The drawing under review shows one solid part. Ordinate dimensions are in mm from its lowest x, y, z. A direction names the side the tool comes from. Coordinates: 2 decimals unless noted, no trailing zeros. Write each loop counter-clockwise with the first axis right and the second up, starting at its lowest first coordinate (ties: lowest second). Pieces come first, ordered by that corner, then holes. Notation, with made-up numbers: (16, -9) - (28, -9) arc R28 ccw to (28, 18) - close; hole circle Ø9 at (49, 34.25). An arc over 180 degrees is marked (long way). Put each result on its own line as item: value. Start each with the question number.
Item 1: Mouldability with a two-part tool opening along X and no side actions: class the marked faces 1, 2, 3 and 4 as pulls with the +X half, pulls with the -X half, needs draft (parallel to the pull), parting line crosses it, or undercut.
Item 2: Consider section A-A on x = 10. Give the boundary of the cut face in (y, z), then the cut area to 3 significant figures.
Item 3: For pin 1 (2 mm diameter, centred on x = 14.5, y = 3.5, fed in from -Z); pin 2 (12 mm diameter, centred on y = 16.5, z = 20.5, fed in from -X); pin 3 (12 mm diameter, centred on x = 10, z = 22.5, fed in from +Y), all flat-tipped, find the tip position at first contact; note any pin that passes through.
Item 4: Consider section D-D on z = 20.5. Give the boundary of the cut face in (x, y), then the cut area to 4 significant figures.
Item 5: Consider section C-C on y = 12.5. Give the boundary of the cut face in (x, z), then the cut area to 3 significant figures.
Item 6: Consider section B-B on z = 4.25. Give the boundary of the cut face in (x, y), then the cut area to 3 significant figures.
Item 7: To check wall thickness, follow L1, parallel to Z at x = 12.5, y = 10; L2, parallel to X at y = 10, z = 4.5; L3, parallel to Z at x = 17.5, y = 7.75. State the ranges of each line that lie inside material, in increasing order. Write a range as [from, to].
Item 8: Machinability: for the marked faces 5, 6, 7, 8 and 9, which of the approach directions +Z, -Z, +X, -X, +Y, -Y give a long, thin tool a straight path to every point of the face, cutting with its end or side? Answer none if there is none.
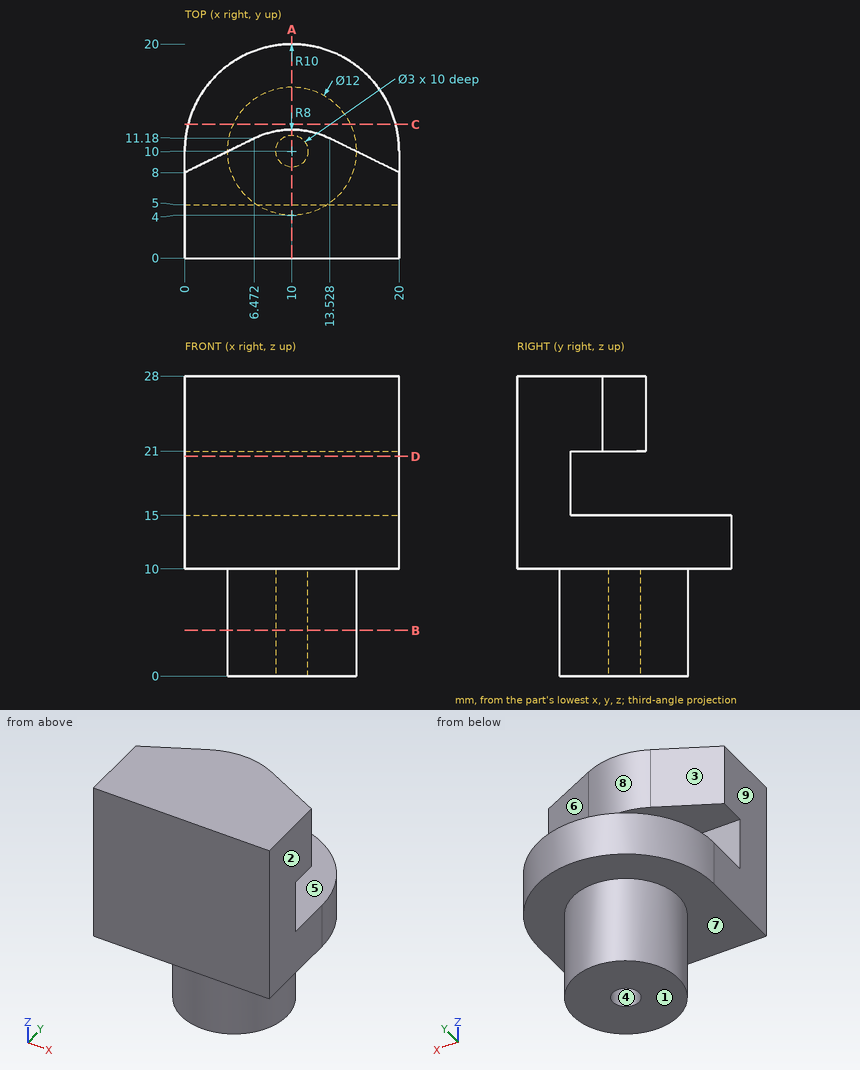
Report:
1. face 1: needs draft
1. face 2: pulls with the +X half
1. face 3: pulls with the -X half
1. face 4: undercut
2. outline: (0, 10) - (4, 10) - (4, 0) - (8.5, 0) - (8.5, 10) - (11.5, 10) - (11.5, 0) - (16, 0) - (16, 10) - (20, 10) - (20, 15) - (5, 15) - (5, 21) - (12, 21) - (12, 28) - (0, 28) - close
2. area: 304 mm²
3. pin 1: z = 10
3. pin 2: x = 0.88
3. pin 3: y = 12
4. outline: (0, 0) - (20, 0) - (20, 5) - (0, 5) - close
4. area: 100.0 mm²
5. outline: (0.32, 10) - (4.55, 10) - (4.55, 0) - (15.45, 0) - (15.45, 10) - (19.68, 10) - (19.68, 15) - (0.32, 15) - close
5. area: 206 mm²
6. outline: circle Ø12 at (10, 10); hole circle Ø3 at (10, 10)
6. area: 106 mm²
7. L1: [0, 15], [21, 28]
7. L2: [4, 8.5], [11.5, 16]
7. L3: [10, 15], [21, 28]
8. face 5: +X, -X, +Y
8. face 6: +Z, +X, +Y
8. face 7: -Z
8. face 8: +Z, +Y
8. face 9: +Z, -Z, -X, +Y, -Y
